```python
from build123d import *

# Parameters (mm, degrees)
SKETCH_1_W               = 30
SKETCH_1_H               = 30
SKETCH_1_R               = 1.5
EXTRUDE_1_DEPTH          = 3
SKETCH_2_W               = 30
SKETCH_2_H               = 2
EXTRUDE_2_DEPTH          = 18
CUT_EXTRUDE_1_DEPTH      = 39.078865529
CUT_EXTRUDE_1_DEPTH_BACK = 39.078865529
SKETCH_3_R               = 1.5
CUT_EXTRUDE_2_DEPTH      = 40.572717875
FILLET_1_R               = 2


with BuildPart() as part:
    # 草图1 → 凸台-拉伸1 (new body)
    with BuildSketch(Plane.XY):
        Rectangle(SKETCH_1_W, SKETCH_1_H)
        with Locations((-10, 10)):
            Circle(SKETCH_1_R, mode=Mode.SUBTRACT)
        with Locations((10, 10)):
            Circle(SKETCH_1_R, mode=Mode.SUBTRACT)
        with Locations((-10, -10)):
            Circle(SKETCH_1_R, mode=Mode.SUBTRACT)
        with Locations((10, -10)):
            Circle(SKETCH_1_R, mode=Mode.SUBTRACT)
    extrude(amount=EXTRUDE_1_DEPTH)

    # 草图2 → 凸台-拉伸2 (add)
    with BuildSketch(Plane.XY.offset(3)):
        with Locations((0, 14)):
            Rectangle(SKETCH_2_W, SKETCH_2_H)
        with Locations((0, -14)):
            Rectangle(SKETCH_2_W, SKETCH_2_H)
    extrude(amount=EXTRUDE_2_DEPTH)

    # 草图3 → 切除-拉伸1 (cut, two sides: drawn at the far end of the back side and taken through both)
    with BuildSketch(Plane.XZ.offset(-13).offset(-CUT_EXTRUDE_1_DEPTH_BACK)):
        with Locations((-11, 10)):
            Circle(SKETCH_3_R)
        with Locations(Location((11, 10, 0), (0, 0, 270))):
            Circle(SKETCH_3_R)
    extrude(amount=CUT_EXTRUDE_1_DEPTH + CUT_EXTRUDE_1_DEPTH_BACK, mode=Mode.SUBTRACT)

    # 草图4 → 切除-拉伸2 (cut, through all)
    with BuildSketch(Plane.XZ.offset(15)):
        with BuildLine():
            Line((-7, 13), (-16.491106969, 13))
            Line((-16.491106969, 13), (-16.491106969, 22.234658659))
            Line((-16.491106969, 22.234658659), (16.365937277, 22.234658659))
            Line((16.365937277, 22.234658659), (16.365937277, 13))
            Line((16.365937277, 13), (7, 13))
            ThreePointArc((7, 13), (0, 6), (-7, 13))
        make_face()
    extrude(amount=-CUT_EXTRUDE_2_DEPTH, mode=Mode.SUBTRACT)

    # 圆角1
    fillet_1_edges = [part.edges().sort_by_distance(p)[0] for p in [
        (7, 14, 13),
        (7, -14, 13),
        (-15, 14, 13),
        (-7, 14, 13),
        (-15, -14, 13),
        (-7, -14, 13),
        (15, 14, 13),
        (15, -14, 13),
    ]]
    fillet(fillet_1_edges, radius=FILLET_1_R)


solid = part.part
```
Here's how the part is built. I have some questions about the finished solid (model axes, mm). A direction names the side the tool comes from. Round coordinates to 2 decimals unless told otherwise and drop trailing zeros. Order: outer loops, then holes, each group sorted by start corner. A loop starts at its lowest first (then second) coordinate and runs counter-clockwise, first axis right, second up. Notation, with made-up numbers: M 1.25,-14 L 31.25,-14 A9 cw 31.25,-4 Z; hole C 59.25,5 d5. An arc over 180 degrees is marked long. Answer in a Markdown table with one row per item.
Item 1: I'm going to push flat-ended pins straight in: pin 1 (5 mm diameter, centred on x = 4.5, z = 8, fed in from +Y); pin 2 (8 mm diameter, centred on x = -1.5, y = 4.5, fed in from +Z). Where does each tip first touch, or does it pass through?
A:
| item | result |
|---|---|
| pin 1 | stops at y = 15 |
| pin 2 | stops at z = 3 |
Item 2: For faces 4 (the face through (-7.543, 14.014, 12.575)), 5 (the face through (8.8, 9.1, 1.5)), 6 (the face through (-0.2, 13, 5.7)), which set-ups out of +Z, -Z, +X, -X, +Y, -Y let a thin tool reach every point of the face, with its end or its side?
A:
| item | result |
|---|---|
| face 4 | +Z, +Y, -Y |
| face 5 | +Z, -Z |
| face 6 | +Z, +X, -X |
Item 3: Imagine slicing it at A-A, the plane z = 5.25. Write out the boundary of the cut face in (x, y), and give its area (3 significant figures).
A:
| item | result |
|---|---|
| outline | M -15,-15 L 15,-15 L 15,-13 L -15,-13 Z; M -15,13 L 15,13 L 15,15 L -15,15 Z |
| area | 120 mm2 |
Item 4: Imagine slicing it at B-B, the plane y = -10. Write out the boundary of the cut face in (x, z).
A:
| item | result |
|---|---|
| outline | M -15,0 L -11.5,0 L -11.5,3 L -15,3 Z; M -8.5,0 L 8.5,0 L 8.5,3 L -8.5,3 Z; M 11.5,0 L 15,0 L 15,3 L 11.5,3 Z |
Item 5: If I drill on L1, parallel to Y at x = -10, z = 0.6; L2, parallel to Y at x = -7.75, z = 9.75; L3, parallel to Z at x = 11, y = -14.25, over which ranges is the centre line in solid material (lowest first)? Write a range as from..to.
A:
| item | result |
|---|---|
| L1 | y = -15..-11.5, -8.5..8.5, 11.5..15 |
| L2 | y = -15..-13, 13..15 |
| L3 | z = 0..8.5, 11.5..13 |
Item 6: Imagine slicing it at C-C, the plane x = 11. Write out the boundary of the cut face in (y, z).
A:
| item | result |
|---|---|
| outline | M -15,0 L -11.12,0 L -11.12,3 L -13,3 L -13,8.5 L -15,8.5 Z; M -15,11.5 L -13,11.5 L -13,13 L -15,13 Z; M -8.88,0 L 8.88,0 L 8.88,3 L -8.88,3 Z; M 11.12,0 L 15,0 L 15,8.5 L 13,8.5 L 13,3 L 11.12,3 Z; M 13,11.5 L 15,11.5 L 15,13 L 13,13 Z |
Item 7: Imagine slicing it at D-D, the plane z = 7. Write out the boundary of the cut face in (x, y).
A:
| item | result |
|---|---|
| outline | M -15,-15 L -3.61,-15 L -3.61,-13 L -15,-13 Z; M -15,13 L -3.61,13 L -3.61,15 L -15,15 Z; M 3.61,-15 L 15,-15 L 15,-13 L 3.61,-13 Z; M 3.61,13 L 15,13 L 15,15 L 3.61,15 Z |
Item 8: Thinking about a two-plate mould opening in X: for faces 1 (the face through (7.543, -13.986, 12.575)), 2 (the face through (0, 15, 5)), 3 (the face through (-14.43, -13.99, 12.4)), which applies, +X half, -X half, draft (parallel to the pull), parting line (faces both ways), or undercut?
A:
| item | result |
|---|---|
| face 1 | undercut |
| face 2 | draft |
| face 3 | -X half |
